Could you check a few things on this model? Use its own coordinates, in mm. Give positions to 0.01 mm unless a question says otherwise; leave off trailing zeros. Loops run counter-clockwise (first coordinate to the right, second up) from the corner with the lowest first, then second, coordinate; pieces in that order, holes last. Notation, with made-up numbers: (30.5, 70) - (84.5, 70) arc R6 cw to (84.5, 79) - close; hole circle Ø5 at (64, 0.25). An arc over 180 degrees is marked (long way). Write each question's results on one line, items separated by ' | '. Start each with the question number.
1) I want a section at A-A, the plane x = 0. Write out the boundary of the cut face in (y, z), and give its area (3 significant figures).
2) If I drill on probe 1 along Y at (x, z) = (0.5, 155); probe 2 along X at (y, z) = (-2, 428); probe 3 along Y at (x, z) = (21.5, 308.5), over which ranges is the centre line in solid material (lowest first)? Write a range as [from, to].
3) I'm going to push flat-ended pins straight in: pin 1 (3 mm diameter, centred on y = -22, z = 720.5, fed in from +X); pin 2 (1 mm diameter, centred on x = -6, z = 558.5, fed in from -Y); pin 3 (4 mm diameter, centred on x = 10, z = 654.5, fed in from +Y). Where does each tip first touch, or does it pass through?
4) I want a section at B-B, the plane y = 0. Write out the boundary of the cut face in (x, z).
5) I want a section at C-C, the plane z = 104. Write out the boundary of the cut face in (x, y), and give its area (3 significant figures).
from build123d import *

# Parameters (mm, degrees)
SKETCH1_R           = 30
BOSS_EXTRUDE2_DEPTH = 830
CUT_EXTRUDE4_DEPTH  = 70
CUT_EXTRUDE5_DEPTH  = 70


with BuildPart() as part:
    # Sketch1 → Boss-Extrude2 (new body)
    with BuildSketch(Plane.XY):
        Circle(SKETCH1_R)
    extrude(amount=BOSS_EXTRUDE2_DEPTH)

    # Sketch3 → Cut-Extrude4 (cut)
    with BuildSketch(Plane(origin=(0, 40, 0), x_dir=(1, 0, 0), z_dir=(0, 1, 0))):
        Polygon((-30, 0), (30, -60), (30, 0), align=None)
    extrude(amount=-CUT_EXTRUDE4_DEPTH, mode=Mode.SUBTRACT)

    # Sketch4 → Cut-Extrude5 (cut)
    with BuildSketch(Plane(origin=(0, 40, 0), x_dir=(1, 0, 0), z_dir=(0, 1, 0))):
        Polygon((-30, -830), (30, -830), (30, -770), align=None)
    extrude(amount=-CUT_EXTRUDE5_DEPTH, mode=Mode.SUBTRACT)


solid = part.part
Answers:
1) outline: (-30, 30) - (30, 30) - (30, 800) - (-30, 800) - close | area: 46,200 mm2
2) probe 1: y = [-30, 30] | probe 2: x = [-29.93, 29.93] | probe 3: y = [-20.92, 20.92]
3) pin 1: stops at x = 21.9 | pin 2: stops at y = -29.49 | pin 3: stops at y = 28.91
4) outline: (-30, 0) - (30, 60) - (30, 770) - (-30, 830) - close
5) outline: circle Ø60 at (0, 0) | area: 2,830 mm2
